Verification items for the finished model (mm, model axes). A direction names the side the tool comes from. Give positions to 0.01 mm unless a question says otherwise; leave off trailing zeros. Write each loop counter-clockwise with the first axis right and the second up, starting at its lowest first coordinate (ties: lowest second). Pieces come first, ordered by that corner, then holes. Notation, with made-up numbers: M -37.75,-1.75 L 3.25,-1.75 A15 ccw 3.25,22.25 Z; hole C 14,-12.75 d1. An arc over 180 degrees is marked long. Write item = value, one per line.
from build123d import *

# Parameters (mm, degrees)
SKETCH028_R     = 1.5
PAD012_DEPTH    = 3
SKETCH029_R     = 9
SKETCH030_R     = 5
PAD018_DEPTH    = 6
POCKET002_DEPTH = 5
FILLET001_R     = 1
SKETCH052_W     = 8
SKETCH052_H     = 8
SKETCH051_W     = 8
SKETCH051_H     = 8
SKETCH053_R     = 1.5
POCKET003_DEPTH = 15
POCKET004_DEPTH = 2.5
POCKET005_DEPTH = 2


with BuildPart() as part:
    # Sketch028 (on Face1 of Binder008) → Pad012 (new body)
    with BuildSketch(Plane(origin=(-61, 0, 0), x_dir=(0, -1, 0), z_dir=(-1, 0, 0))):
        with BuildLine():
            Line((-21.15, 15.5), (-21.15, -134.35))
            ThreePointArc((-21.15, -134.35), (-19.495153, -138.345153), (-15.5, -140))
            Line((-15.5, -140), (15.5, -140))
            ThreePointArc((15.5, -140), (19.495153, -138.345153), (21.15, -134.35))
            Line((21.15, 15.5), (21.15, -134.35))
            ThreePointArc((21.15, 15.5), (19.495153, 19.495153), (15.5, 21.15))
            Line((-15.5, 21.15), (15.5, 21.15))
            ThreePointArc((-15.5, 21.15), (-19.495153, 19.495153), (-21.15, 15.5))
        make_face()
        with Locations((15.5, -134.35)):
            Circle(SKETCH028_R, mode=Mode.SUBTRACT)
        with Locations((-15.5, -134.35)):
            Circle(SKETCH028_R, mode=Mode.SUBTRACT)
        with BuildLine():
            ThreePointArc((17, -31.15), (15.5, -29.65), (14, -31.15))
            Line((14, -31.15), (14, -129.35))
            ThreePointArc((14, -129.35), (15.5, -130.85), (17, -129.35))
            Line((17, -129.35), (17, -31.15))
        make_face(mode=Mode.SUBTRACT)
        with BuildLine():
            ThreePointArc((-14, -31.15), (-15.5, -29.65), (-17, -31.15))
            Line((-17, -31.15), (-17, -129.35))
            ThreePointArc((-17, -129.35), (-15.5, -130.85), (-14, -129.35))
            Line((-14, -129.35), (-14, -31.15))
        make_face(mode=Mode.SUBTRACT)
        with BuildLine():
            ThreePointArc((-2.2, -1.65), (2.75, 0), (-2.2, 1.65))
            Line((-2.2, 1.65), (-2.2, -1.65))
        make_face(mode=Mode.SUBTRACT)
    extrude(amount=PAD012_DEPTH)

    # Sketch029 (on Face21 of Pad012) → AdditiveLoft002 section 0
    with BuildSketch(Plane.YZ.offset(-61)):
        Circle(SKETCH029_R)
    # Sketch030 (on Face21 of Pad012) → AdditiveLoft002 section 1
    with BuildSketch(Plane.YZ.offset(-45)):
        Circle(SKETCH030_R)
    loft()

    # Sketch033 (on Face21 of Pad012) → SubtractiveLoft section 0
    with BuildSketch(Plane.YZ.offset(-61)):
        with BuildLine():
            ThreePointArc((2.2, 1.65), (-2.75, 0), (2.2, -1.65))
            Line((2.2, 1.65), (2.2, -1.65))
        make_face()
    # Sketch032 (on Binder) → SubtractiveLoft section 1
    with BuildSketch(Plane.YZ.offset(-45)):
        with BuildLine():
            ThreePointArc((2.2, 1.65), (-2.75, 0), (2.2, -1.65))
            Line((2.2, 1.65), (2.2, -1.65))
        make_face()
    loft(mode=Mode.SUBTRACT)

    # Sketch041 (on Face4 of SubtractiveLoft) → Pad018 (join)
    with BuildSketch(Plane.YZ.offset(-61)):
        with BuildLine():
            ThreePointArc((3, 11.783809), (0, 12.159693), (-3, 11.783809))
            Line((-3, 11.783809), (-3, 2.75))
            Line((-3, 2.75), (3, 2.75))
            Line((3, 11.783809), (3, 2.75))
        make_face()
    extrude(amount=PAD018_DEPTH)

    # Sketch042 (on Face28 of Pad018) → Pocket002 (cut)
    with BuildSketch(Plane.YZ.offset(-55)):
        with BuildLine():
            Line((-2.05, 10.985643), (2.05, 10.985643))
            Line((2.05, 10.985643), (2.05, 11.985643))
            ThreePointArc((2.05, 11.985643), (0, 12.159693), (-2.05, 11.985643))
            Line((-2.05, 10.985643), (-2.05, 11.985643))
        make_face()
    extrude(amount=-POCKET002_DEPTH, mode=Mode.SUBTRACT)

    # Fillet001
    fillet001_edges = [part.edges().sort_by_distance(p)[0] for p in [
        (-55, -3, 9.328836),
        (-55, 3, 9.328836),
    ]]
    fillet(fillet001_edges, radius=FILLET001_R)

    # Sketch052 (on Face7 of Fillet001) → AdditiveLoft003 section 0
    with BuildSketch(Plane.YZ.offset(-45)):
        with Locations((6.2, 0)):
            Rectangle(SKETCH052_W, SKETCH052_H)
    # Sketch051 (on Face4 of Fillet001) → AdditiveLoft003 section 1
    with BuildSketch(Plane.YZ.offset(-61)):
        with Locations((6.2, 0)):
            Rectangle(SKETCH051_W, SKETCH051_H)
    loft()

    # Sketch053 (on Face39 of AdditiveLoft003) → Pocket003 (cut)
    with BuildSketch(Plane.XZ.offset(-2.2)):
        with Locations((-50, 0)):
            Circle(SKETCH053_R)
    extrude(amount=-POCKET003_DEPTH, mode=Mode.SUBTRACT)

    # Sketch054 (on Face40 of Pocket003) → Pocket004 (cut)
    with BuildSketch(Plane.XZ.offset(-2.2)):
        Polygon((-51.645448, 2.85), (-53.290897, 0), (-51.645448, -2.85), (-48.354552, -2.85), (-45, -2.85), (-45, 2.85), (-48.354552, 2.85), align=None)
    extrude(amount=-POCKET004_DEPTH, mode=Mode.SUBTRACT)

    # Sketch055 (on Face33 of Pocket004) → Pocket005 (cut)
    with BuildSketch(Plane(origin=(0, 10.2, 0), x_dir=(-1, 0, 0), z_dir=(0, 1, 0))):
        with BuildLine():
            ThreePointArc((50, -2.6), (52.6, 0), (50, 2.6))
            Line((50, 2.6), (45, 2.6))
            Line((45, 2.6), (45, -2.6))
            Line((45, -2.6), (50, -2.6))
        make_face()
    extrude(amount=-POCKET005_DEPTH, mode=Mode.SUBTRACT)


solid = part.part
1) Tool access check on faces 1 (the cylindrical face through (-62.48, 15.47, -29.65)), 2 (the flat face through (-51, 7, 4)), 3 (the cylindrical face through (-51.5, 6.43, 0.07)). Record the directions out of +Z, -Z, +X, -X, +Y, -Y that give a thin tool (end or side, any length) a straight path to the whole face; none if there is none.
From the geometry:
face_1 = +X, -X
face_2 = +Z, +X, +Y
face_3 = +Y
2) Cross-section at B-B on z = -42. Record the boundary of the cut face in (x, y), plus the area to 3 significant figures.
From the geometry:
outline = M -64,-21.15 L -61,-21.15 L -61,-17 L -64,-17 Z; M -64,-14 L -61,-14 L -61,14 L -64,14 Z; M -64,17 L -61,17 L -61,21.15 L -64,21.15 Z
area = 109 mm^2
3) Depth check by flat-ended pin: P1, Ø1.4, axis at x = -59, z = 9.5, coming from the -Y side; P2, Ø1.5, axis at y = -7.5, z = -96.5, coming from the +X side; P3, Ø0.6, axis at x = -49, z = -2.5, coming from the +Y side. Enter the tip coordinate at first touch or a pass-through.
From the geometry:
P1 = -3
P2 = -61
P3 = 10.2
4) Cross-section at C-C on x = -57.5. Record the boundary of the cut face in (y, z) (3 decimals), plus the area to 3 significant figures.
From the geometry:
outline = M -3,7.551 A8.125 ccw long 7.072,-4 L 10.2,-4 L 10.2,4 L 7.072,4 A8.125 ccw 3,7.551 L 3,11.784 A12.16 ccw 2.05,11.986 L 2.05,10.986 L -2.05,10.986 L -2.05,11.986 A12.16 ccw -3,11.784 Z; hole M 2.2,-1.65 L 2.2,1.65 A2.75 ccw long Z
area = 224 mm^2
5) Cross-section at A-A on y = 0. Record the boundary of the cut face in (x, z).
From the geometry:
outline = M -64,-140 L -61,-140 L -61,-9 L -45,-5 L -45,-2.75 L -64,-2.75 Z; M -64,2.75 L -45,2.75 L -45,5 L -55,7.5 L -55,10.99 L -60,10.99 L -60,12.16 L -61,12.16 L -61,21.15 L -64,21.15 Z
6) Draft check along Z on faces 4 (the flat face through (-55, 0, 9)), 5 (the flat face through (-62, 0, -140)), 6 (the flat face through (-62, -14, -80)). Enter one of: +Z half, -Z half, draft (parallel to the pull), parting line (faces both ways), or undercut.
From the geometry:
face_4 = draft
face_5 = -Z half
face_6 = undercut
7) Cross-section at D-D on z = -16. Record the boundary of the cut face in (x, y), plus the area to 3 significant figures.
From the geometry:
outline = M -64,-21.15 L -61,-21.15 L -61,21.15 L -64,21.15 Z
area = 127 mm^2
8) Material ranges on probe 1 along Y at (x, z) = (-62.5, -119.5); probe 2 along Z at (x, y) = (-50, 5.65); probe 3 along Z at (x, y) = (-63.3, 0), recorded low to high. Write a range as from..to.
From the geometry:
probe_1 = -21.15..-17, -14..14, 17..21.15
probe_2 = -4..-1.5, 1.5..4
probe_3 = -140..-2.75, 2.75..21.15
